```python
from build123d import *

# Parameters (mm, degrees)
SKETCH1_W           = 61
SKETCH1_H           = 61
BOSS_EXTRUDE1_DEPTH = 1.6
SKETCH2_W           = 15
SKETCH2_H           = 15
BOSS_EXTRUDE2_DEPTH = 4.8


with BuildPart() as part:
    # Sketch1 → Boss-Extrude1 (new body)
    with BuildSketch(Plane(origin=(0, 0, 0), x_dir=(1, 0, 0), z_dir=(0, 1, 0))):
        Rectangle(SKETCH1_W, SKETCH1_H)
    extrude(amount=BOSS_EXTRUDE1_DEPTH)

    # Sketch2 → Boss-Extrude2 (add)
    with BuildSketch(Plane(origin=(0, 1.6, 0), x_dir=(1, 0, 0), z_dir=(0, 1, 0))):
        with Locations((-19, 19)):
            Rectangle(SKETCH2_W, SKETCH2_H)
        with Locations((0, 19)):
            Rectangle(SKETCH2_W, SKETCH2_H)
        with Locations((19, 19)):
            Rectangle(SKETCH2_W, SKETCH2_H)
        with Locations((19, 0)):
            Rectangle(SKETCH2_W, SKETCH2_H)
        Rectangle(SKETCH2_W, SKETCH2_H)
        with Locations((-19, 0)):
            Rectangle(SKETCH2_W, SKETCH2_H)
        with Locations((-19, -19)):
            Rectangle(SKETCH2_W, SKETCH2_H)
        with Locations((0, -19)):
            Rectangle(SKETCH2_W, SKETCH2_H)
        with Locations((19, -19)):
            Rectangle(SKETCH2_W, SKETCH2_H)
    extrude(amount=BOSS_EXTRUDE2_DEPTH)


solid = part.part
```
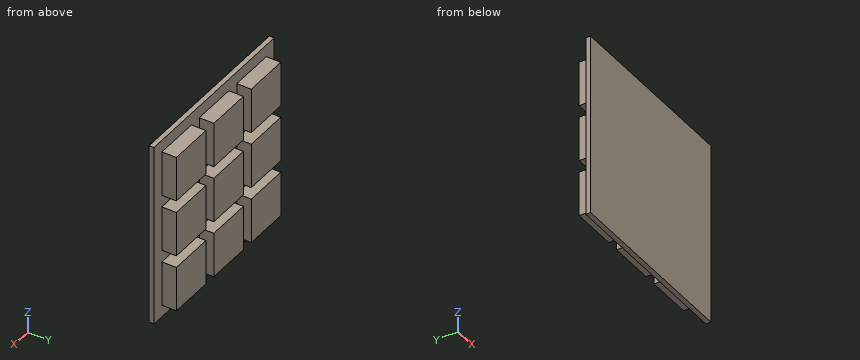
For this review, take the finished solid that the model builds, in its own axes (mm). Coordinates: 2 decimals unless noted, no trailing zeros. Loops run counter-clockwise (first coordinate to the right, second up) from the corner with the lowest first, then second, coordinate; pieces in that order, holes last. Notation, with made-up numbers: (-11.75, -34.75) -> (33.25, -34.75) arc R18 cw to (33.25, -30.75) -> close; hole circle Ø10 at (-14, 45.5). An arc over 180 degrees is marked (long way). Return JSON: item names as keys, results as strings. Group by question number.
(1) Consider section A-A, the plane z = 1. Give the boundary of the cut face in (x, y).
(2) Consider section B-B, the plane x = 2.5. Give the boundary of the cut face in (y, z).
(3) For pin 1 Ø2.5 at (y, z) = (3, -20.5) entering from +X; pin 2 Ø3 at (x, y) = (-4, 4) entering from +Z; pin 3 Ø1.4 at (y, z) = (3, -16) entering from -X, all flat-tipped, find the tip position at first contact; note any pin that passes through.
(4) To check wall thickness, follow L1, parallel to X at y = 2, z = 0.5; L2, parallel to Y at x = 6, z = 8. State the ranges of each line that lie inside material, in increasing order.
(5) Consider section C-C, the plane y = 2.5. Count the separate pieces of the cut face and the enclosed holes in it, plus the area to 4 significant figures.
(6) Consider section D-D, the plane z = 8.5. Give the boundary of the cut face in (x, y), plus the area to 3 significant figures.
Results below:
{
 "1": {"outline": "(-30.5, 0) -> (30.5, 0) -> (30.5, 1.6) -> (26.5, 1.6) -> (26.5, 6.4) -> (11.5, 6.4) -> (11.5, 1.6) -> (7.5, 1.6) -> (7.5, 6.4) -> (-7.5, 6.4) -> (-7.5, 1.6) -> (-11.5, 1.6) -> (-11.5, 6.4) -> (-26.5, 6.4) -> (-26.5, 1.6) -> (-30.5, 1.6) -> close"},
 "2": {"outline": "(0, -30.5) -> (1.6, -30.5) -> (1.6, -26.5) -> (6.4, -26.5) -> (6.4, -11.5) -> (1.6, -11.5) -> (1.6, -7.5) -> (6.4, -7.5) -> (6.4, 7.5) -> (1.6, 7.5) -> (1.6, 11.5) -> (6.4, 11.5) -> (6.4, 26.5) -> (1.6, 26.5) -> (1.6, 30.5) -> (0, 30.5) -> close"},
 "3": {"pin 1": "stops at x = 26.5", "pin 2": "stops at z = 26.5", "pin 3": "stops at x = -26.5"},
 "4": {"L1": "x = -26.5 to -11.5, -7.5 to 7.5, 11.5 to 26.5", "L2": "y = 0 to 1.6"},
 "5": {"separate pieces": "9", "enclosed holes": "0", "area": "2,025 mm2"},
 "6": {"outline": "(-30.5, 0) -> (30.5, 0) -> (30.5, 1.6) -> (-30.5, 1.6) -> close", "area": "97.6 mm2"}
}
